The drawing under review shows one solid part. Ordinate dimensions are in mm from its lowest x, y, z. Give positions to 0.01 mm unless a question says otherwise; leave off trailing zeros. Write each loop counter-clockwise with the first axis right and the second up, starting at its lowest first coordinate (ties: lowest second). Pieces come first, ordered by that corner, then holes. Notation, with made-up numbers: (18, 22.25) -> (39, 22.25) arc R32 ccw to (39, 48.25) -> close; hole circle Ø1 at (12, -31.5). An arc over 180 degrees is marked (long way). Use CSV: the item, a comma, the result in double quotes.
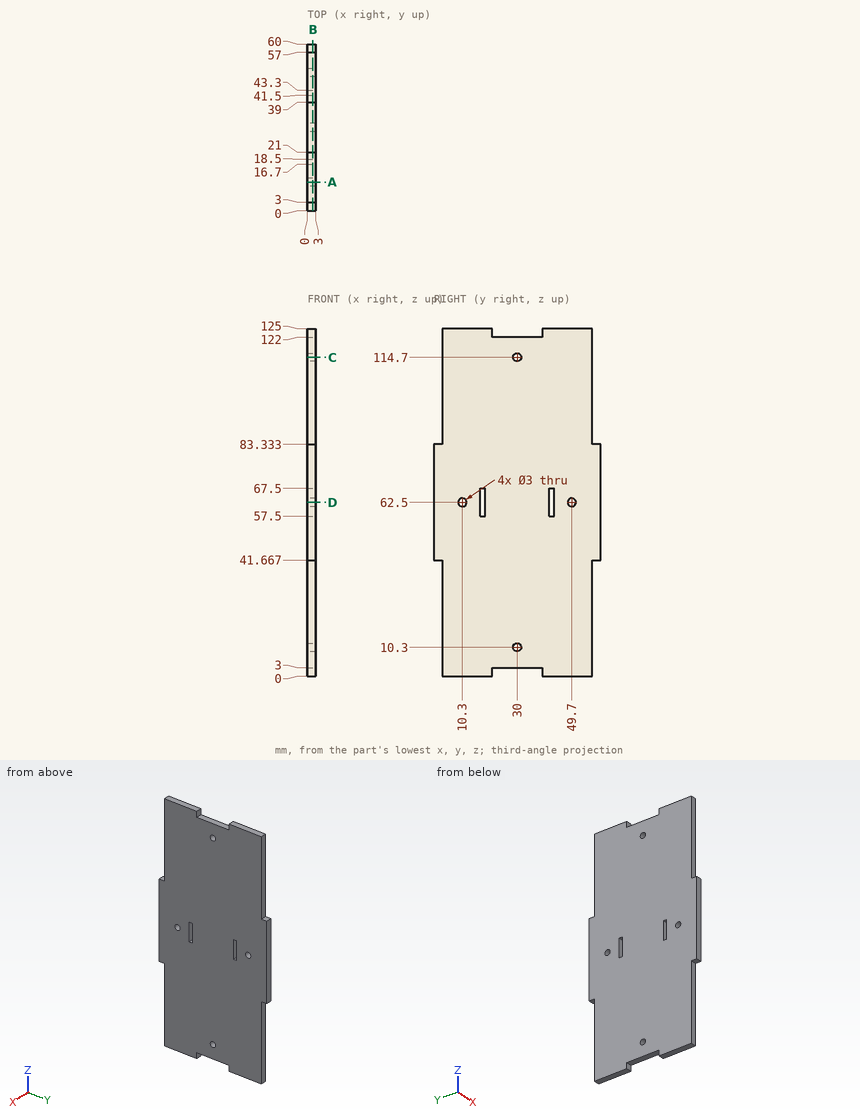
(1) Take a section at D-D (z = 62.5). Write out the cut boundary in (x, y), then the cut area to 3 significant figures.
Established:
outline,"(0, 0) -> (3, 0) -> (3, 8.8) -> (0, 8.8) -> close; (0, 11.8) -> (3, 11.8) -> (3, 16.7) -> (0, 16.7) -> close; (0, 18.5) -> (3, 18.5) -> (3, 41.5) -> (0, 41.5) -> close; (0, 43.3) -> (3, 43.3) -> (3, 48.2) -> (0, 48.2) -> close; (0, 51.2) -> (3, 51.2) -> (3, 60) -> (0, 60) -> close"
area,"151 mm2"
(2) Take a section at A-A (y = 10.3). Write out the cut boundary in (x, z), then the cut area to 3 significant figures.
Established:
outline,"(0, 0) -> (3, 0) -> (3, 61) -> (0, 61) -> close; (0, 64) -> (3, 64) -> (3, 125) -> (0, 125) -> close"
area,"366 mm2"
(3) For line 1 along Z through (x, y) = (0.85, 29.5) (1 decimal); line 2 along Z through (x, y) = (2.1, 18); line 3 along Y through (x, z) = (0.75, 108), list the stretches that pass through material, from the lowest coordinate up. Write a range as [from, to].
Established:
line 1,"z = [3, 8.9], [11.7, 113.3], [116.1, 122]"
line 2,"z = [0, 57.5], [67.5, 125]"
line 3,"y = [3, 57]"
(4) Take a section at B-B (x = 1.9). State how many separate pieces and enclosed holes the cut face has, then the cut area to 3 significant figures.
Established:
separate pieces,"1"
enclosed holes,"6"
area,"6,830 mm2"
(5) Clearance check with flat-ended pins moving along their axes: pin 1 (0.9 mm diameter, centred on x = 1.5, z = 124, fed in from +Y); pin 2 (0.9 mm diameter, centred on x = 1, y = 30.5, fed in from +Z); pin 3 (1.5 mm diameter, centred on x = 1, y = 26.5, fed in from -Z). State where each tip first meets the part, or that it passes through.
Established:
pin 1,"stops at y = 57"
pin 2,"stops at z = 122"
pin 3,"stops at z = 3"
(6) Take a section at C-C (z = 114.7). Write out the cut boundary in (x, y).
Established:
outline,"(0, 3) -> (3, 3) -> (3, 28.5) -> (0, 28.5) -> close; (0, 31.5) -> (3, 31.5) -> (3, 57) -> (0, 57) -> close"
